Can you work these out from the model? Positions are in its coordinate system, mm. A direction names the side the tool comes from. Give positions to 0.01 mm unless a question says otherwise; leave off trailing zeros. Loops run counter-clockwise (first coordinate to the right, second up) from the corner with the lowest first, then second, coordinate; pieces in that order, holes last. Notation, with made-up numbers: (65, 38.25) -> (118, 38.25) arc R31 cw to (118, 77.25) -> close; hole circle Ø8 at (6.5, 2). An arc over 180 degrees is marked (long way). Return JSON: item names as keys, results as strings. Group by question number.
Q1. Thinking about a two-plate mould opening in Y: for faces 1 (the cylindrical face through (2.98, -26.53, 8.93)), 2 (the flat face through (-1.75, -16, 7)), 3 (the cylindrical face through (-4.596, -6.581, 7.395)), 4 (the cylindrical face through (0.242, 7.496, 7.395)), which applies, pulls with the +Y half, pulls with the -Y half, needs draft (parallel to the pull), parting line crosses it, or undercut?
Q2. Suppose I cut it at A-A, the plane y = -22. Please give me the cut outline in (x, z).
Q3. Suppose I cut it at C-C, the plane z = 7.5. Please give me the cut outline in (x, y) (3 decimals), and give its area (3 significant figures).
Q4. I need wall thicknesses on line 1 along Z through (x, y) = (3.65, -22); line 2 along X through (y, z) = (0, 7.25); line 3 along X through (y, z) = (-10, 11.5). Which ranges of each line are inside material? Lowest first, please. Write a range as [from, to].
Q5. Will these pins go through, and if not, where does the flat tip stop? pin 1 (7.5 mm diameter, centred on y = -19, z = 10, fed in from -X); pin 2 (7.5 mm diameter, centred on y = -22, z = 7.5, fed in from +X); pin 3 (7.5 mm diameter, centred on y = -14.5, z = 4, fed in from +X); pin 4 (2 mm diameter, centred on x = 4.5, z = 8, fed in from +Y).
Q6. Suppose I cut it at B-B, the plane y = -10. Please give me the cut outline in (x, z).
Q7. Which directions (+Z, -Z, +X, -X, +Y, -Y) give clear straight access to the entire face, cutting with the end or side of a thin tool? Please do faces 5 (the flat face through (-4.25, -17, 7)), 6 (the flat face through (4.25, -17, 7)), 7 (the flat face through (1.75, -16, 7)), 8 (the flat face through (3, -30, 7)), 9 (the flat face through (-2, -11, 0)).
Q8. Suppose I cut it at D-D, the plane x = 3. Please give me the cut outline in (y, z), and give its area (3 significant figures).
```python
from build123d import *

# Parameters (mm, degrees)
F1_DEPTH = 15
F3_D     = 9.5


with BuildPart() as f1:
    # F0 (on Top) → F1 (new body)
    with BuildSketch(Plane.XY):
        with BuildLine():
            ThreePointArc((-3.375, -3.689089), (0, 5), (3.375, -3.689089))
            ThreePointArc((3.375, -3.689089), (2.174249, -5.362613), (1.75, -7.378177))
            Line((1.75, -7.378177), (1.75, -30))
            Line((1.75, -30), (4.25, -30))
            Line((4.25, -30), (4.25, -8.407586))
            ThreePointArc((4.25, -8.407586), (4.58631, -6.60481), (5.55, -5.044552))
            ThreePointArc((5.55, -5.044552), (0, 7.5), (-5.55, -5.044552))
            ThreePointArc((-5.55, -5.044552), (-4.58631, -6.60481), (-4.25, -8.407586))
            Line((-4.25, -8.407586), (-4.25, -30))
            Line((-4.25, -30), (-1.75, -30))
            Line((-1.75, -30), (-1.75, -7.378177))
            ThreePointArc((-1.75, -7.378177), (-2.174249, -5.362613), (-3.375, -3.689089))
        make_face()
    extrude(amount=F1_DEPTH)

    # F3 (through all)
    with Locations(Plane.YZ.offset(4.25)):
        with Locations((-22, 7.5)):
            Hole(F3_D / 2)


solid = f1.part
```
Ans:
{
 "1": {"face 1": "undercut", "face 2": "needs draft", "face 3": "pulls with the -Y half", "face 4": "parting line crosses it"},
 "2": {"outline": "(-4.25, 0) -> (-1.75, 0) -> (-1.75, 2.75) -> (-4.25, 2.75) -> close; (-4.25, 12.25) -> (-1.75, 12.25) -> (-1.75, 15) -> (-4.25, 15) -> close; (1.75, 0) -> (4.25, 0) -> (4.25, 2.75) -> (1.75, 2.75) -> close; (1.75, 12.25) -> (4.25, 12.25) -> (4.25, 15) -> (1.75, 15) -> close"},
 "3": {"outline": "(-5.55, -5.045) arc R5 cw to (-4.25, -8.408) -> (-4.25, -17.25) -> (-1.75, -17.25) -> (-1.75, -7.378) arc R5 ccw to (-3.375, -3.689) arc R5 cw (long way) to (3.375, -3.689) arc R5 ccw to (1.75, -7.378) -> (1.75, -17.25) -> (4.25, -17.25) -> (4.25, -8.408) arc R5 cw to (5.55, -5.045) arc R7.5 ccw (long way) to start; (-4.25, -30) -> (-1.75, -30) -> (-1.75, -26.75) -> (-4.25, -26.75) -> close; (1.75, -30) -> (4.25, -30) -> (4.25, -26.75) -> (1.75, -26.75) -> close", "area": "157 mm^2"},
 "4": {"line 1": "z = [0, 2.75], [12.25, 15]", "line 2": "x = [-7.5, -5], [5, 7.5]", "line 3": "x = [-4.25, -1.75], [1.75, 4.25]"},
 "5": {"pin 1": "stops at x = -4.25", "pin 2": "passes through", "pin 3": "stops at x = 4.25", "pin 4": "stops at y = 6.63"},
 "6": {"outline": "(-4.25, 0) -> (-1.75, 0) -> (-1.75, 15) -> (-4.25, 15) -> close; (1.75, 0) -> (4.25, 0) -> (4.25, 15) -> (1.75, 15) -> close"},
 "7": {"face 5": "+Z, -Z, -X, -Y", "face 6": "+Z, -Z, +X, -Y", "face 7": "+Z, -Z, -Y", "face 8": "+Z, -Z, +X, -X, -Y", "face 9": "-Z, +X, -X, +Y, -Y"},
 "8": {"outline": "(-30, 0) -> (-4.07, 0) -> (-4.07, 15) -> (-30, 15) -> close; (4, 0) -> (6.87, 0) -> (6.87, 15) -> (4, 15) -> close; hole circle Ø9.5 at (-22, 7.5)", "area": "361 mm^2"}
}
